Check sheet for the drawn part. Datum: minimum x, y, z corner. Units: mm. A direction names the side the tool comes from. Give positions to 0.01 mm unless a question says otherwise; leave off trailing zeros. Loops run counter-clockwise (first coordinate to the right, second up) from the corner with the lowest first, then second, coordinate; pieces in that order, holes last. Notation, with made-up numbers: M -0.5,40 L 36.5,40 A30 cw 36.5,69 Z; hole C 88,84 d4. An arc over 180 degrees is marked long. Write each question's results on one line, items separated by ' | '. Start each with the question number.
1. Tool access check on the marked faces 4, 5 and 6. Record the directions out of +Z, -Z, +X, -X, +Y, -Y that give a thin tool (end or side, any length) a straight path to the whole face; none if there is none.
2. Go/stop test with flat-tipped pins: pin 1 (5 mm diameter, centred on y = 17.5, z = 1.5, fed in from +X); pin 2 (2.5 mm diameter, centred on x = 5, z = 5, fed in from +Y); pin 3 (5 mm diameter, centred on x = 51, z = 5.5, fed in from +Y). Record where each tip stops, or that it passes through.
3. Material ranges on line 1 along Z through (x, y) = (5, 1.3); line 2 along Y through (x, z) = (30, 5.25) (1 decimal); line 3 along X through (y, z) = (14.5, 2.5), recorded low to high.
4. Sectioned sample at B-B on z = 5. Give the number of separate pieces and of enclosed holes in the cut face.
5. Sectioned sample at C-C on y = 33.5. Record the cut outline in (x, z), and give its area (3 significant figures).
6. Sectioned sample at A-A on x = 55. Record the cut outline in (y, z).
7. Draft check along Y on the marked faces 1, 2 and 3. Enter one of: pulls with the +Y half, pulls with the -Y half, needs draft (parallel to the pull), parting line crosses it, or undercut.
8. Sectioned sample at D-D on x = 15. Record the cut outline in (y, z).
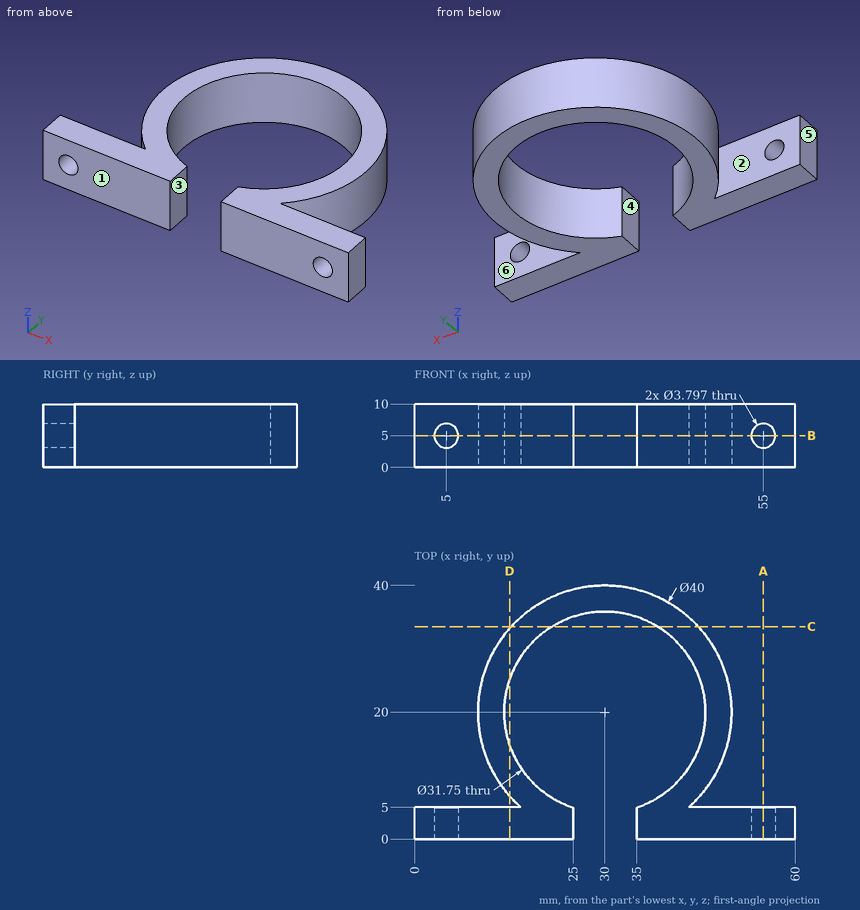
Output values:
1) face 4: +Z, -Z, -Y | face 5: +Z, -Z, -X, +Y, -Y | face 6: +Z, -Z, +X
2) pin 1: x = 50 | pin 2: through | pin 3: y = 27.6
3) line 1: 0 to 3.1, 6.9 to 10 | line 2: 35.9 to 40 | line 3: 10.77 to 15.11, 44.89 to 49.23
4) separate pieces: 3 | enclosed holes: 0
5) outline: M 15.24,0 L 21.65,0 L 21.65,10 L 15.24,10 Z; M 38.35,0 L 44.76,0 L 44.76,10 L 38.35,10 Z | area: 128 mm2
6) outline: M 0,0 L 5,0 L 5,3.1 L 0,3.1 Z; M 0,6.9 L 5,6.9 L 5,10 L 0,10 Z
7) face 1: pulls with the -Y half | face 2: undercut | face 3: needs draft
8) outline: M 0,0 L 5,0 L 5,10 L 0,10 Z; M 6.77,0 L 14.8,0 L 14.8,10 L 6.77,10 Z; M 25.2,0 L 33.23,0 L 33.23,10 L 25.2,10 Z
